Could you check a few things on this model? Use its own coordinates, in mm. Give positions to 0.01 mm unless a question says otherwise; leave off trailing zeros. Loops run counter-clockwise (first coordinate to the right, second up) from the corner with the lowest first, then second, coordinate; pieces in that order, holes last. Notation, with made-up numbers: (41, -6) - (72, -6) arc R15 cw to (72, 13) - close; hole circle Ø8 at (20.5, 1). An arc over 180 degrees is marked (long way). Use CSV: the item, a comma, the result in double quotes.
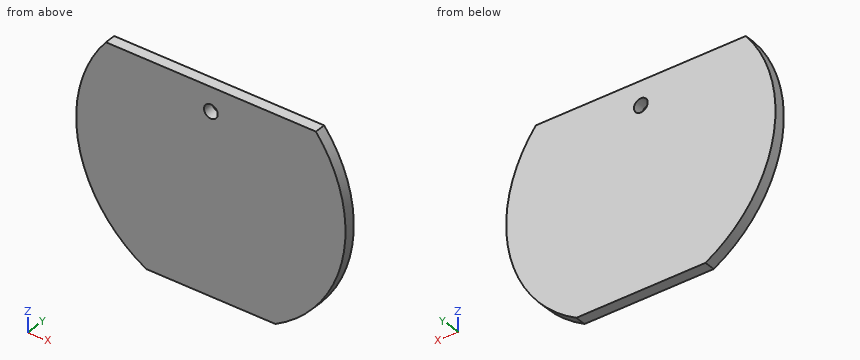
Autodesk Inventor part; units mm, degrees
ref_plane "YZ Plane" through (0, 0, 0) normal (1, 0, 0) x (0, 1, 0)
ref_plane "XZ Plane" through (0, 0, 0) normal (0, 1, 0) x (-1, 0, 0)
ref_plane "XY Plane" through (0, 0, 0) normal (0, 0, 1) x (1, 0, 0)
sketch "スケッチ1" plane through (0, 0, 0) normal (0, 1, 0) x (-1, 0, 0)
  point P0 (0, 0)
sketch "スケッチ2" plane through (0, 0, 0) normal (0, 1, 0) x (-1, 0, 0)
  arc A0 (-19.1073, 15.335) -> (-11.7473, -21.5) centre (0, 0) ccw
  line L0 (0, 0) -> (0, -21.5)
  line L1 (0, 0) -> (0, 15.335)
  line L2 (0, -21.5) -> (-11.7473, -21.5)
  line L3 (0, 15.335) -> (-19.1073, 15.335)
  dimension "d1" = 21.5
  dimension "d3" = 15.335
  dimension "d4" = 24.5
extrude "押し出し1" add sketch "スケッチ2" along normal blind 2
sketch "スケッチ3" plane through (0, 2, 0) normal (0, 1, 0) x (1, 0, 0)
  line L0 (0, 21.5) -> (0, -15.335)
  circle A0 centre (0, -11) radius 1.25
  point P0 (0, 0)
  point P1 (0, -9.75)
  point P2 (0, -12.25)
  dimension "d7" = 2.5
  dimension "d8" = 11
extrude "押し出し2" cut sketch "スケッチ3" against normal blind 10 contours A0 L0 picked at (0.1808, -10.6246)
mirror "ミラー2" about plane through (0, 0, -21.5) normal (-1, 0, 0) of "押し出し2", "押し出し1"
properties part number "huta"
1) Suppose I cut it at C-C (z = 10.5). Please give me the cut outline in (x, y).
Answer below:
outline,"(-22.14, 0) - (-1.15, 0) - (-1.15, 2) - (-22.14, 2) - close; (1.15, 0) - (22.14, 0) - (22.14, 2) - (1.15, 2) - close"
2) I need wall thicknesses on line 1 along Z through (x, y) = (0, 1.1) (3 decimals); line 2 along X through (y, z) = (0.5, 11); line 3 along Z through (x, y) = (-14, 0.2) (3 decimals). Which ranges of each line are inside material? Lowest first, please.
Answer below:
line 1,"z = -21.5 to 9.75, 12.25 to 15.335"
line 2,"x = -21.89 to -1.25, 1.25 to 21.89"
line 3,"z = -20.106 to 15.335"
3) Suppose I cut it at A-A (x = 0). Please give me the cut outline in (y, z) (3 decimals), plus the area to 3 significant figures.
Answer below:
outline,"(0, -21.5) - (2, -21.5) - (2, 9.75) - (0, 9.75) - close; (0, 12.25) - (2, 12.25) - (2, 15.335) - (0, 15.335) - close"
area,"68.7 mm2"
4) Suppose I cut it at B-B (y = 1.4). Please give me the cut outline in (x, z) (3 decimals).
Answer below:
outline,"(-19.107, 15.335) arc R24.5 ccw to (-11.747, -21.5) - (11.747, -21.5) arc R24.5 ccw to (19.107, 15.335) - close; hole circle Ø2.5 at (0, 11)"
5) Suppose I cut it at D-D (z = -9.5). Please give me the cut outline in (x, y).
Answer below:
outline,"(-22.58, 0) - (22.58, 0) - (22.58, 2) - (-22.58, 2) - close"
6) I'm going to push flat-ended pins straight in: P1, Ø10, axis at x = -15.5, z = -10.5, coming from the -Y side; P2, Ø1, axis at y = 0.5, z = -8, coming from the -X side; P3, Ø1.5, axis at x = 0, z = 11, coming from the +Y side. Where does each tip first touch, or does it pass through?
Answer below:
P1,"stops at y = 0"
P2,"stops at x = -23.32"
P3,"passes through"
